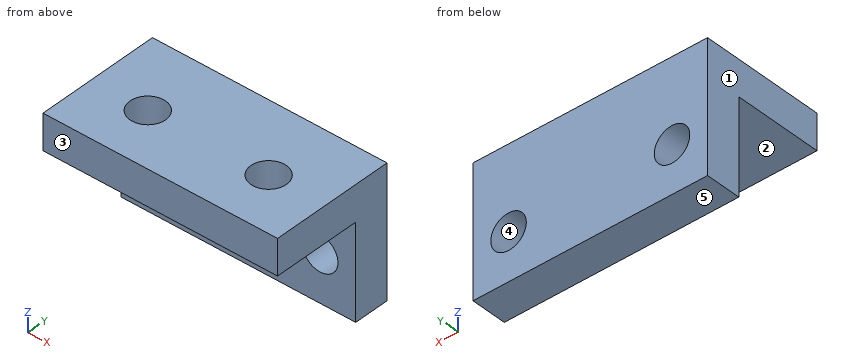
```python
from build123d import *

# Parameters (mm, degrees)
SKETCH_W        = 19.8
SKETCH_H        = 14.5
SKETCH_R        = 1.5
PAD_DEPTH       = 3
SKETCH001_W     = 19.8
SKETCH001_H     = 3
PAD001_DEPTH    = 8
SKETCH002_R     = 1.5
POCKET_DEPTH    = 3.001
SKETCH003_W     = 4
SKETCH003_H     = 3
POCKET001_DEPTH = 19.801


with BuildPart() as part:
    # Sketch → Pad (new body)
    with BuildSketch(Plane.XY):
        with Locations((9.9, 7.25)):
            Rectangle(SKETCH_W, SKETCH_H)
        with Locations((4.8, 8.6)):
            Circle(SKETCH_R, mode=Mode.SUBTRACT)
        with Locations((15, 8.6)):
            Circle(SKETCH_R, mode=Mode.SUBTRACT)
    extrude(amount=PAD_DEPTH)

    # Sketch001 → Pad001 (new body)
    with BuildSketch(Plane(origin=(0, 0, 0), x_dir=(1, 0, 0), z_dir=(0, 0, -1))):
        with Locations((9.9, -13)):
            Rectangle(SKETCH001_W, SKETCH001_H)
    extrude(amount=PAD001_DEPTH)

    # Sketch002 → Pocket (cut, through all)
    with BuildSketch(Plane.XZ.offset(-11.5)):
        with Locations((3, -4)):
            Circle(SKETCH002_R)
        with Locations((16.8, -4)):
            Circle(SKETCH002_R)
    extrude(amount=-POCKET_DEPTH, mode=Mode.SUBTRACT)

    # Sketch003 → Pocket001 (cut, through all)
    with BuildSketch(Plane.YZ.offset(19.8)):
        with Locations((2, 1.5)):
            Rectangle(SKETCH003_W, SKETCH003_H)
    extrude(amount=-POCKET001_DEPTH, mode=Mode.SUBTRACT)


solid = part.part
```
Geometry: final body of the model. Coordinates: model frame, mm. Face numbers are marked on the shaded views. A direction names the side the tool comes from. Round coordinates to 2 decimals unless told otherwise and drop trailing zeros. Loops run counter-clockwise (first coordinate to the right, second up) from the corner with the lowest first, then second, coordinate; pieces in that order, holes last. Notation, with made-up numbers: (68.25, 70) -> (94.25, 70) arc R22 ccw to (94.25, 106) -> close; hole circle Ø9 at (-19, 56). An arc over 180 degrees is marked (long way). Use one line per item in the form item = value. Start each with the question number.
1) Section B-B on z = -4. Output: boundary loops of the cut face in (x, y).
2) Section A-A on x = 4.8. Output: boundary loops of the cut face in (y, z).
3) Draft query along Z for the marked faces 3, 4 and 5. Return one class per face: released by +Z, released by -Z, zero draft, split by the parting line, or undercut.
4) First-contact query: P1, Ø2.5, axis at x = 16.8, z = -4, coming from the +Y side; P2, Ø6.5, axis at x = 8.5, z = -2.5, coming from the -Y side; P3, Ø3, axis at x = 5.5, y = 9.5, coming from the -Z side. Flat tips, straight axial feed; report the tip coordinate or a pass-through.
5) Section C-C on y = 8.6. Output: boundary loops of the cut face in (x, z), then the cut area to 3 significant figures.
6) Line query: L1, parallel to Y at x = 4.8, z = 1.7; L2, parallel to Z at x = 3, y = 12.8; L3, parallel to X at y = 11.75, z = -3.5. Output: solid intervals per line, ascending.
7) Access query for the marked faces 1 and 2. Directions: +Z, -Z, +X, -X, +Y, -Y. A direction counts if a zero-diameter tool reaches every point of the face in a straight line with its end or side. Return the directions, or none.
8) Section D-D on y = 11.75. Output: boundary loops of the cut face in (x, z), then the cut area to 3 significant figures.
Response:
q1.outline = (0, 11.5) -> (1.5, 11.5) -> (1.5, 14.5) -> (0, 14.5) -> close; (4.5, 11.5) -> (15.3, 11.5) -> (15.3, 14.5) -> (4.5, 14.5) -> close; (18.3, 11.5) -> (19.8, 11.5) -> (19.8, 14.5) -> (18.3, 14.5) -> close
q2.outline = (4, 0) -> (7.1, 0) -> (7.1, 3) -> (4, 3) -> close; (10.1, 0) -> (11.5, 0) -> (11.5, -8) -> (14.5, -8) -> (14.5, 3) -> (10.1, 3) -> close
q3.face_3 = zero draft
q3.face_4 = undercut
q3.face_5 = released by -Z
q4.P1 = through
q4.P2 = 4
q4.P3 = 0
q5.outline = (0, 0) -> (3.3, 0) -> (3.3, 3) -> (0, 3) -> close; (6.3, 0) -> (13.5, 0) -> (13.5, 3) -> (6.3, 3) -> close; (16.5, 0) -> (19.8, 0) -> (19.8, 3) -> (16.5, 3) -> close
q5.area = 41.4 mm^2
q6.L1 = 4 to 7.1, 10.1 to 14.5
q6.L2 = -8 to -5.5, -2.5 to 3
q6.L3 = 0 to 1.59, 4.41 to 15.39, 18.21 to 19.8
q7.face_1 = +Z, -Z, -X, +Y, -Y
q7.face_2 = -Z, +X, -X, -Y
q8.outline = (0, -8) -> (19.8, -8) -> (19.8, 3) -> (0, 3) -> close; hole circle Ø3 at (3, -4); hole circle Ø3 at (16.8, -4)
q8.area = 204 mm^2
